Could you check a few things on this model? Use its own coordinates, in mm. A direction names the side the tool comes from. Round coordinates to 2 decimals unless told otherwise and drop trailing zeros. Order: outer loops, then holes, each group sorted by start corner. A loop starts at its lowest first (then second) coordinate and runs counter-clockwise, first axis right, second up. Notation, with made-up numbers: M 61.5,24 L 102.5,24 A28 cw 102.5,60 Z; hole C -1,29 d8. An arc over 180 degrees is marked long. Write each question's results on one line, items separated by ' | '. Start each with the question number.
1. I'm going to push flat-ended pins straight in: pin 1 (5 mm diameter, centred on y = -18, z = -22, fed in from +X); pin 2 (4 mm diameter, centred on x = 27.5, y = -18.5, fed in from +Z); pin 3 (12 mm diameter, centred on x = 76.5, y = -24.5, fed in from -Z). Where does each tip first touch, or does it pass through?
2. For faces 1 (the flat face through (67.734, -37.567, -37.529)), 2 (the flat face through (8.08, -37.57, 16.89)), 3 (the flat face through (41, -76.2, -14)), which set-ups out of +Z, -Z, +X, -X, +Y, -Y let a thin tool reach every point of the face, with its end or its side?
3. We'd pull the mould along X, two halves only. Please class faces 4 (the flat face through (-11.64, -37.57, 7.98)), 5 (the flat face through (41, 0, -14)), 6 (the flat face through (111.43, -37.57, -35.71)): released by +X, released by -X, zero draft, split by the parting line, or undercut.
4. Suppose I cut it at C-C on x = 28. Write out the boundary of the cut face in (y, z).
5. Please list where these lines run through material, in increasing order: L1, parallel to X at y = -60.5, z = 9; L2, parallel to X at y = -55, z = 6; L3, parallel to Z at x = -11, y = -19.
6. Suppose I cut it at D-D on z = -29. Write out the boundary of the cut face in (x, y).
7. Suppose I cut it at B-B on y = -68.5. Write out the boundary of the cut face in (x, z), and give its area (3 significant figures).
8. Suppose I cut it at A-A on z = 7. Write out the boundary of the cut face in (x, y).
from build123d import *

# Parameters (mm, degrees)
F1_DEPTH = 76.2
F2_DEPTH = 76.2


with BuildPart() as f1:
    # F0 (on Front) → F1 (new body)
    with BuildSketch(Plane.XZ):
        Polygon((15.9395597875, 33.3230420947), (0, 0), (-23.6055366695, 16.1788745644), (-23.6055366695, -36.3934971392), (33.8444890328, -21.3188421257), (51.7809395939, 16.1788745644), align=None)
    extrude(amount=F1_DEPTH)

    # F2 (add): a face of the model
    f2_faces = [f1.faces().sort_by_distance(p)[0] for p in [
        (42.8127143134, -38.1, -2.5699837806),
    ]]
    extrude(f2_faces, amount=F2_DEPTH)


solid = f1.part
Filled sheet:
1) pin 1: stops at x = 119.18 | pin 2: stops at z = 28.75 | pin 3: stops at z = -44.59
2) face 1: -Z, +Y, -Y | face 2: +Z, +Y, -Y | face 3: +Z, -Z, +X, -X, -Y
3) face 4: undercut | face 5: zero draft | face 6: released by +X
4) outline: M -76.2,-22.85 L 0,-22.85 L 0,27.55 L -76.2,27.55 Z
5) L1: x = -23.61 to -13.13, 4.31 to 66.79 | L2: x = -23.61 to -8.75, 2.87 to 73.06 | L3: z = -33.09 to 7.54
6) outline: M -23.61,-76.2 L 4.57,-76.2 L 4.57,0 L -23.61,0 Z; M 49.9,-76.2 L 114.64,-76.2 L 114.64,0 L 49.9,0 Z
7) outline: M -23.61,-36.39 L 33.84,-21.32 L 102.59,-54.2 L 120.52,-16.7 L 15.94,33.32 L 0,0 L -23.61,16.18 Z | area: 6,210 mm^2
8) outline: M -23.61,-76.2 L -10.21,-76.2 L -10.21,0 L -23.61,0 Z; M 3.35,-76.2 L 70.97,-76.2 L 70.97,0 L 3.35,0 Z
